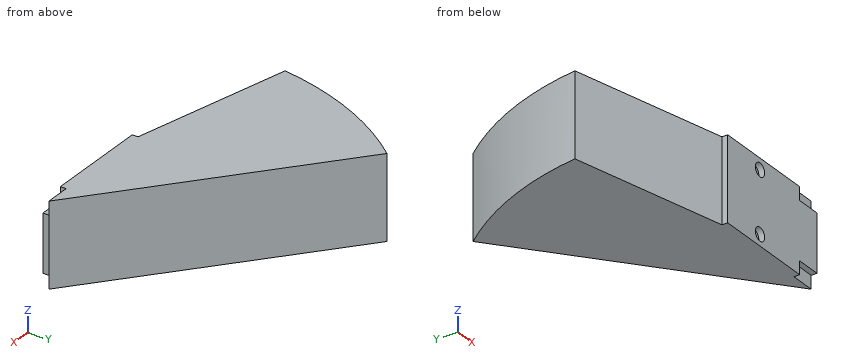
```python
from build123d import *

# Parameters (mm, degrees)
SKETCH1_R           = 4.566693037
SKETCH1_W           = 17.1
SKETCH1_H           = 39.4
BOSS_EXTRUDE1_DEPTH = 4
BOSS_EXTRUDE2_REACH = 107.531


with BuildPart() as part:
    # Sketch1 → Boss-Extrude1 (new body)
    # profile 1 of 2: a face of its own
    with BuildSketch(Plane(origin=(0, 0, 0), x_dir=(1, 0, 0), z_dir=(0, 1, 0))):
        Polygon((0, 57.5), (0, 0), (71.3, 0), (71.3, 9.05), (71.3, 48.45), (71.3, 57.5), align=None)
        with Locations(Location((31.977132175, 7.725129874, 0), (0, 0, 270))):
            Circle(SKETCH1_R, mode=Mode.SUBTRACT)
        with Locations(Location((31.977132175, 49.774870126, 0), (0, 0, 270))):
            Circle(SKETCH1_R, mode=Mode.SUBTRACT)
    # profile 2 of 2: a face of its own
    with BuildSketch(Plane(origin=(0, 0, 0), x_dir=(1, 0, 0), z_dir=(0, 1, 0))):
        with Locations((79.85, 28.75)):
            Rectangle(SKETCH1_W, SKETCH1_H)
    extrude(amount=BOSS_EXTRUDE1_DEPTH)

    # Boss-Extrude2: up to this face of the body (flat: up to its plane)
    boss_extrude2_end = Plane(part.part.faces().sort_by_distance((35.65, 2, -57.5))[0])
    # Sketch2 → Boss-Extrude2 (add, up to the picked face)
    with BuildSketch(Plane.XY, mode=Mode.PRIVATE) as boss_extrude2_sk1:
        with BuildLine():
            Line((0, 4), (88.4, 4))
            Line((88.4, 4), (-64.878686432, 130.222546803))
            ThreePointArc((-64.878686432, 130.222546803), (-93.746808792, 83.050787997), (-108.484737296, 29.746596971))
            Line((-108.484737296, 29.746596971), (0, 4))
        make_face()
    boss_extrude2_tool1 = split(extrude(boss_extrude2_sk1.sketch, amount=-BOSS_EXTRUDE2_REACH, mode=Mode.PRIVATE), bisect_by=boss_extrude2_end, keep=Keep.BOTH, mode=Mode.PRIVATE)
    add(boss_extrude2_tool1.solids().sort_by(Axis((-29.138762, 51.950808, 0), (0, 0, -1)))[0])


solid = part.part
```
The model under review builds one solid part; all positions refer to its coordinate system, in mm. Round coordinates to 2 decimals unless told otherwise and drop trailing zeros. Loops run counter-clockwise (first coordinate to the right, second up) from the corner with the lowest first, then second, coordinate; pieces in that order, holes last. Notation, with made-up numbers: M 39,5.25 L 43,5.25 A27 cw 43,21.25 Z; hole C 35,-2 d11. An arc over 180 degrees is marked long. Write item = value, one per line.
Item 1: Take a section at B-B on x = 76. Write out the cut boundary in (y, z).
Return value:
outline = M 0,-48.45 L 4,-48.45 L 4,-57.5 L 14.21,-57.5 L 14.21,0 L 4,0 L 4,-9.05 L 0,-9.05 Z
Item 2: Insertion check: P1, Ø2, axis at x = -26.5, z = -43.5, coming from the -Y side; P2, Ø4.5, axis at x = 82.5, z = -3.5, coming from the -Y side; P3, Ø3, axis at y = 1, z = -4, coming from the +X side. Each pin has a flat end and moves straight along its axis. Give the tip position at first contact, or say it passes through.
Return value:
P1 = 10.05
P2 = 4
P3 = 71.3
Item 3: Take a section at C-C on y = 9. Write out the cut boundary in (x, z), then the cut area to 3 significant figures.
Return value:
outline = M -21.07,-57.5 L 82.33,-57.5 L 82.33,0 L -21.07,0 Z
area = 5,950 mm2
Item 4: For line 1 (Y direction, x = 80.5, z = -40.5); line 2 (Y direction, x = 25, z = -37); line 3 (X direction, y = 95.5, z = -2.5), list the stretches that pass through material, from the lowest coordinate up. Write a range as [from, to].
Return value:
line_1 = [0, 10.51]
line_2 = [0, 56.21]
line_3 = [-87.82, -22.71]
Item 5: Take a section at D-D on x = -5.5. Write out the cut boundary in (y, z).
Return value:
outline = M 5.31,-57.5 L 81.33,-57.5 L 81.33,0 L 5.31,0 Z
Item 6: Take a section at A-A on z = -25. Write out the cut boundary in (x, y).
Return value:
outline = M -108.48,29.75 L 0,4 L 0,0 L 88.4,0 L 88.4,4 L -64.88,130.22 A198.56 ccw Z
